For this review, use the dimensioned drawing (mm, ordinates from the lowest corner) and the shaded views. Coordinates: 2 decimals unless noted, no trailing zeros. Loops run counter-clockwise (first coordinate to the right, second up) from the corner with the lowest first, then second, coordinate; pieces in that order, holes last. Notation, with made-up numbers: (58.5, -19.75) - (84.5, -19.75) arc R18 cw to (84.5, 2.25) - close; hole circle Ø7 at (81, 21.25). An arc over 180 degrees is marked (long way). Answer in a Markdown table with one row per item. Add a question column.
(1) To check wall thickness, follow L1, parallel to Y at x = 0.55, z = 9.5; L2, parallel to X at y = 14.75, z = 41; L3, parallel to Z at x = 3.5, y = 14.25. State the ranges of each line that lie inside material, in increasing order. Write a range as [from, to].
(2) We need section D-D, the plane x = 4. Write out the cut boundary in (y, z).
(3) We need section A-A, the plane x = 20. Write out the cut boundary in (y, z).
(4) We need section B-B, the plane y = 10. Write out the cut boundary in (x, z), plus the area to 3 significant figures.
(5) We need section C-C, the plane z = 20. Write out the cut boundary in (x, y).
(6) The part is to be moulded in two halves that separate along Z. For the marked faces 1, 2 and 3, say which applies: released by +Z, released by -Z, zero draft, split by the parting line, or undercut.
(7) Clearance check with flat-ended pins moving along their axes: pin 1 (7 mm diameter, centred on y = 9.5, z = 33.5, fed in from -X); pin 2 (12 mm diameter, centred on y = 14.5, z = 6, fed in from +X); pin 3 (0.6 mm diameter, centred on x = 20, z = 26.5, fed in from +Y). State where each tip first meets the part, or that it passes through.
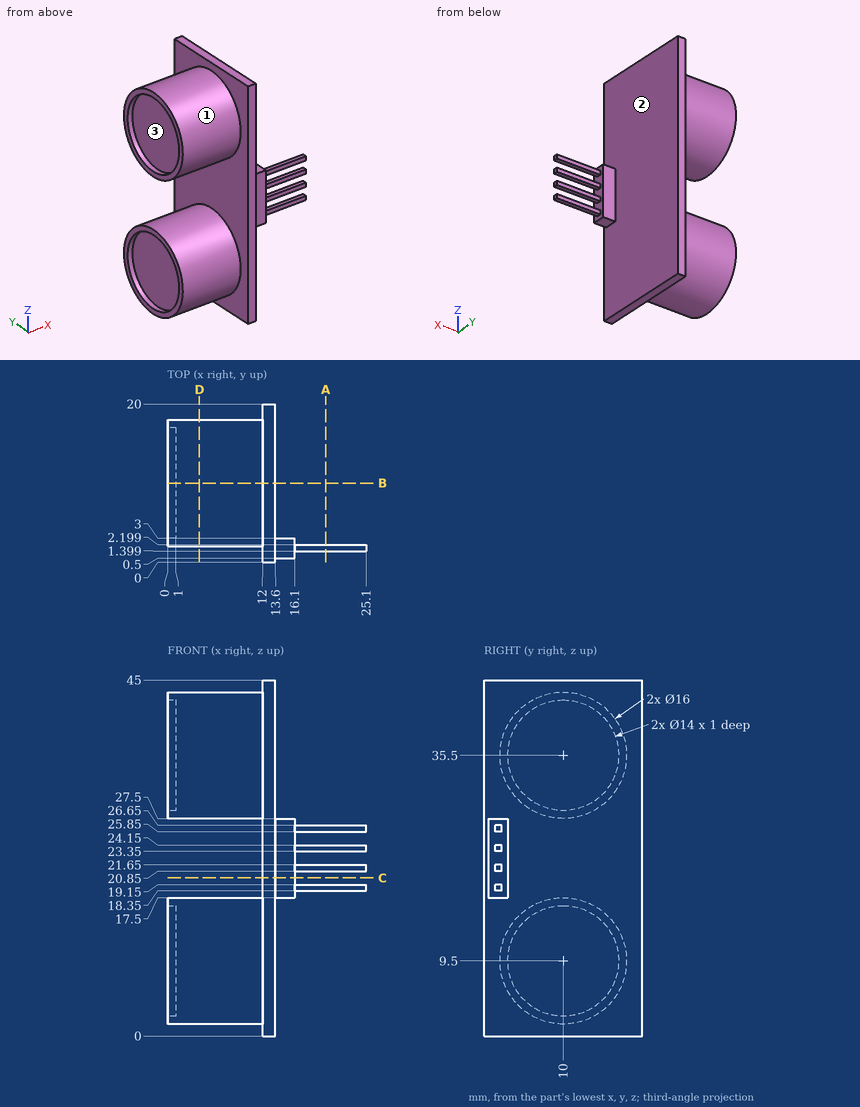
Responses:
| question | item | result |
|---|---|---|
| 1 | L1 | y = [2, 3], [17, 18] |
| 1 | L2 | x = [0, 13.6] |
| 1 | L3 | z = [2.72, 16.28], [28.72, 42.28] |
| 2 | outline | circle Ø16 at (10, 9.5); circle Ø16 at (10, 35.5) |
| 3 | outline | (1.4, 18.35) - (2.2, 18.35) - (2.2, 19.15) - (1.4, 19.15) - close; (1.4, 20.85) - (2.2, 20.85) - (2.2, 21.65) - (1.4, 21.65) - close; (1.4, 23.35) - (2.2, 23.35) - (2.2, 24.15) - (1.4, 24.15) - close; (1.4, 25.85) - (2.2, 25.85) - (2.2, 26.65) - (1.4, 26.65) - close |
| 4 | outline | (0, 1.5) - (12, 1.5) - (12, 0) - (13.6, 0) - (13.6, 45) - (12, 45) - (12, 43.5) - (0, 43.5) - (0, 42.5) - (1, 42.5) - (1, 28.5) - (0, 28.5) - (0, 27.5) - (12, 27.5) - (12, 17.5) - (0, 17.5) - (0, 16.5) - (1, 16.5) - (1, 2.5) - (0, 2.5) - close |
| 4 | area | 428 mm2 |
| 5 | outline | (12, 0) - (13.6, 0) - (13.6, 0.5) - (16.1, 0.5) - (16.1, 3) - (13.6, 3) - (13.6, 20) - (12, 20) - close |
| 6 | face 1 | undercut |
| 6 | face 2 | zero draft |
| 6 | face 3 | undercut |
| 7 | pin 1 | stops at x = 1 |
| 7 | pin 2 | stops at x = 13.6 |
| 7 | pin 3 | stops at y = 2.2 |
